```python
from build123d import *

# Parameters (mm, degrees)
F5_R       = 50
F9_R       = 50
F10_FACE_R = 50
F8_R       = 47.5
F11_FACE_R = 47.5
F7_R       = 50
F12_FACE_R = 50
F6_R       = 50
F14_T      = -1


with BuildPart() as f10:
    # F5 (on offset) → F10 section 0
    with BuildSketch(Plane.XY.offset(50)):
        Circle(F5_R)
    # F9 (on offset) → F10 section 1
    with BuildSketch(Plane.XY.offset(-35)):
        Circle(F9_R)
    loft()

    # F10_face (on face) → F11 section 0
    with BuildSketch(Plane(origin=(0, 0, -35), x_dir=(1, 0, 0), z_dir=(0, 0, -1))):
        Circle(F10_FACE_R)
    # F8 (on offset) → F11 section 1
    with BuildSketch(Plane.XY.offset(-40)):
        Circle(F8_R)
    loft()

    # F11_face (on face) → F12 section 0
    with BuildSketch(Plane(origin=(0, 0, -40), x_dir=(1, 0, 0), z_dir=(0, 0, -1))):
        Circle(F11_FACE_R)
    # F7 (on offset) → F12 section 1
    with BuildSketch(Plane.XY.offset(-45)):
        Circle(F7_R)
    loft()

    # F12_face (on face) → F13 section 0
    with BuildSketch(Plane(origin=(0, 0, -45), x_dir=(1, 0, 0), z_dir=(0, 0, -1))):
        Circle(F12_FACE_R)
    # F6 (on offset) → F13 section 1
    with BuildSketch(Plane.XY.offset(-50)):
        Circle(F6_R)
    loft()

    # F14
    f14_openings = [f10.faces().sort_by_distance(p)[0] for p in [
        (0, 0, 50),
    ]]
    offset(amount=F14_T, openings=f14_openings, kind=Kind.INTERSECTION)


solid = f10.part
```
Model file for the job. Use its own axes, mm. A direction names the side the tool comes from. Coordinates: 2 decimals unless noted, no trailing zeros. Order: outer loops, then holes, each group sorted by start corner. A loop starts at its lowest first (then second) coordinate and runs counter-clockwise, first axis right, second up. Notation, with made-up numbers: (-30, 15) - (2, 15) arc R14 cw to (2, 28) - close; hole circle Ø3 at (-12, 42.5). An arc over 180 degrees is marked (long way). Return JSON: item names as keys, results as strings. Group by question number.
1) Saw through at A-A, the plane z = -12. Write the cut outline in (x, y).
2) Saw through at B-B, the plane x = 0. Write the cut outline in (y, z).
3) Probe line 1 (Y direction, x = 0, z = 13); line 2 (Z direction, x = 29, y = 22); line 3 (Y direction, x = 28.5, z = -38). List the from-to ranges inside material, lowest first. Write a range as from..to.
4) Tool access for faces 1 (the cylindrical face through (26.34, 41.32, 7.02)), 2 (the conical face through (-10.33, 46.52, -40.31)), 3 (the cylindrical face through (47.69, 15.02, 6.91)): list every direction of +Z, -Z, +X, -X, +Y, -Y with a clear straight run to the whole face (end or side of a thin tool).
5) Flat gauge pins, fed straight in: P1, Ø12, axis at x = -2.5, y = 38, coming from the +Z side; P2, Ø2, axis at x = 8.5, z = 1.5, coming from the -Y side; P3, Ø4, axis at x = 29.5, z = 0.5, coming from the -Y side. Where does each tip first touch, or does it go through?
6) Mould opens along X. For faces 4 (the flat face through (-1, 1, -50)), 5 (the cylindrical face through (47.69, -15.02, -47.54)), 6 (the flat face through (-1, 1, -49)) say: released by +X, released by -X, zero draft, split by the parting line, or undercut.
Values found:
{
 "1": {"outline": "circle Ø100 at (0, 0); hole circle Ø98 at (0, 0)"},
 "2": {"outline": "(-50, -50) - (50, -50) - (50, -45) - (47.5, -40) - (50, -35) - (50, 50) - (49, 50) - (49, -34.76) - (46.38, -40) - (49, -45.24) - (49, -49) - (-49, -49) - (-49, -45.24) - (-46.38, -40) - (-49, -34.76) - (-49, 50) - (-50, 50) - (-50, -35) - (-47.5, -40) - (-50, -45) - close"},
 "3": {"line 1": "y = -50..-49, 49..50", "line 2": "z = -50..-49", "line 3": "y = -39.24..-37.85, 37.85..39.24"},
 "4": {"face 1": "+Z", "face 2": "none", "face 3": "+Z, -Z"},
 "5": {"P1": "stops at z = -49", "P2": "stops at y = -49.43", "P3": "stops at y = -41.76"},
 "6": {"face 4": "zero draft", "face 5": "split by the parting line", "face 6": "undercut"}
}
